Input: dimensioned drawing with shaded views. Units: mm. Origin: part minimum x, y, z. A direction names the side the tool comes from. Coordinates: 2 decimals unless noted, no trailing zeros. Write each loop counter-clockwise with the first axis right and the second up, starting at its lowest first coordinate (ties: lowest second). Pieces come first, ordered by that corner, then holes. Notation, with made-up numbers: (-35.5, -23) - (18.5, -23) arc R28 cw to (18.5, -5) - close; hole circle Ø7 at (39, 54.25). An arc over 180 degrees is marked (long way). One line per question, with ' | ' between items.
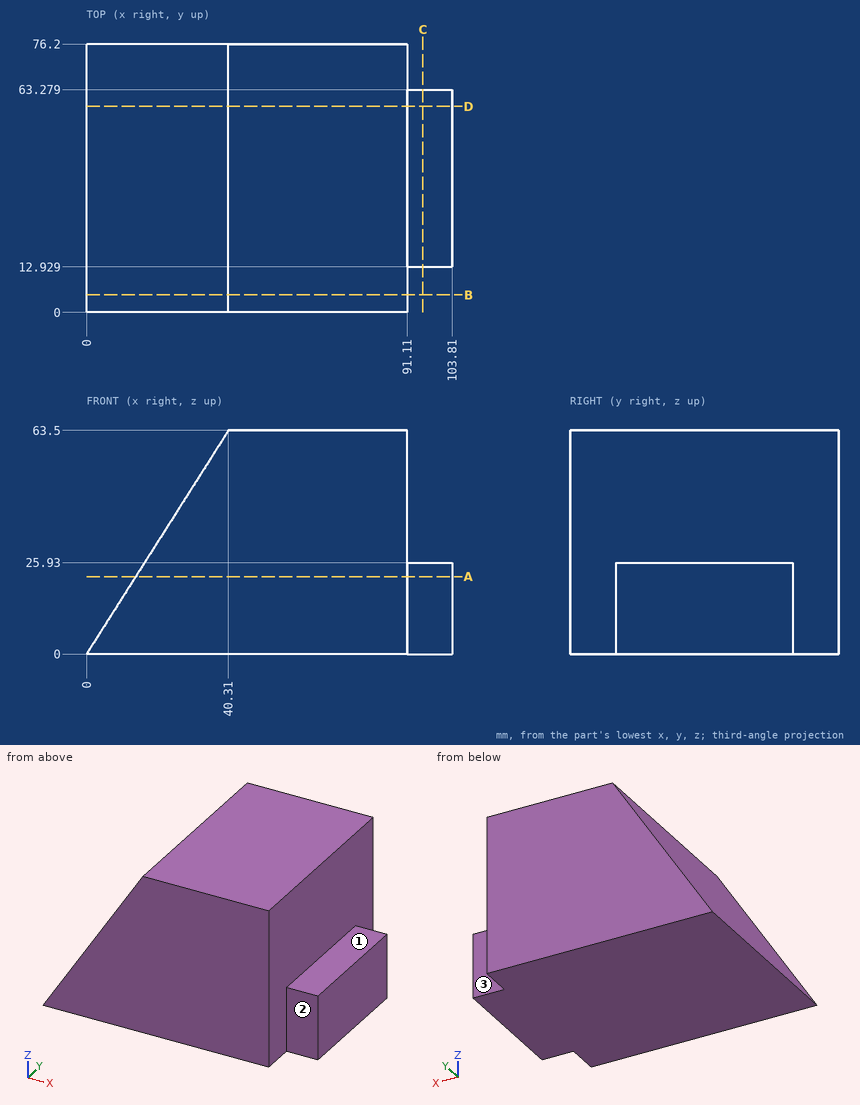
Item 1: Access query for the marked faces 1, 2 and 3. Directions: +Z, -Z, +X, -X, +Y, -Y. A direction counts if a zero-diameter tool reaches every point of the face in a straight line with its end or side. Return the directions, or none.
Check sheet entries:
face 1: +Z, +X, +Y, -Y | face 2: +Z, -Z, +X, -Y | face 3: +Z, -Z, +X, +Y
Item 2: Cut plane D-D on y = 58.5. Return loops of the section in (x, z), and give its area (4 significant figures).
Check sheet entries:
outline: (0, 0) - (103.81, 0) - (103.81, 25.93) - (91.11, 25.93) - (91.11, 63.5) - (40.31, 63.5) - close | area: 4,835 mm²
Item 3: Pin query (flat end, axial travel): pin 1 Ø10 at (x, z) = (98.5, 15) entering from +Y; pin 2 Ø12 at (y, z) = (14.5, 48) entering from -X; pin 3 Ø4 at (x, y) = (94.5, 45.5) entering from +Z. Return the tip coordinate at first contact, or that it passes through.
Check sheet entries:
pin 1: y = 63.28 | pin 2: x = 26.66 | pin 3: z = 25.93
Item 4: Cut plane C-C on x = 95.5. Return loops of the section in (y, z), and give its area (3 significant figures).
Check sheet entries:
outline: (12.93, 0) - (63.28, 0) - (63.28, 25.93) - (12.93, 25.93) - close | area: 1,310 mm²
Item 5: Cut plane A-A on z = 22. Return loops of the section in (x, y) (1 decimal).
Check sheet entries:
outline: (14, 0) - (91.1, 0) - (91.1, 12.9) - (103.8, 12.9) - (103.8, 63.3) - (91.1, 63.3) - (91.1, 76.2) - (14, 76.2) - close
Item 6: Cut plane B-B on y = 5. Return loops of the section in (x, z).
Check sheet entries:
outline: (0, 0) - (91.11, 0) - (91.11, 63.5) - (40.31, 63.5) - close
Item 7: Ray query, line 1 along Y through (x, z) = (98, 14.5); line 2 along Z through (x, y) = (99.5, 23.5); line 3 along X through (y, z) = (70.5, 15). Return the intervals inside material, ascending. Write a range as [from, to].
Check sheet entries:
line 1: [12.93, 63.28] | line 2: [0, 25.93] | line 3: [9.52, 91.11]
